Build history of the part. All positions in model axes, mm. A direction names the side the tool comes from. Give positions to 0.01 mm unless a question says otherwise; leave off trailing zeros. Loops run counter-clockwise (first coordinate to the right, second up) from the corner with the lowest first, then second, coordinate; pieces in that order, holes last. Notation, with made-up numbers: M 66,-37 L 109,-37 A14 cw 109,-23 Z; hole C 50.25,-36.75 d9. An arc over 180 degrees is marked long. Answer as a JSON object with one key per item and string values. Group by question number.
1. Slice it at B-B (x = -0.5). List the corners of the cut face in (y, z), then the cut area to 3 significant figures.
2. Slice it at C-C (y = 65). List the corners of the cut face in (x, z).
3. 3-axis set-ups, long thin cutter, end or side, ignore diameter. For faces 1 (the face through (-13, -1, 0)), 2 (the face through (86.355, 28, 36)): which of +Z, -Z, +X, -X, +Y, -Y reach the whole face in a straight line?
4. Mould opens along Y. For faces 3 (the face through (-109.645, 28, 36)), 4 (the face through (88.355, -4, 35)), 5 (the face through (-13, -102.661, 35)) say: released by +Y, released by -Y, zero draft, split by the parting line, or undercut.
5. Slice it at A-A (z = 32). List the corners of the cut face in (x, y).
6. Drill centre lines: line 1 along Y through (x, z) = (23, 8.5); line 2 along X through (y, z) = (-80, 34); line 3 along X through (y, z) = (42.5, 31). Where is each one in solid material? Low to high. Write a range as [from, to].
7. Drop a flat-ended pin along its axis: pin 1 Ø15 at (x, y) = (-8.5, 24) entering from +Z. Give the stop position or say it passes through.
from build123d import *

# Parameters (mm, degrees)
F0_W     = 200
F0_H     = 200
F1_DEPTH = 70
F2_T     = -2
F3_W     = 196
F3_H     = 2
F3_W_2   = 2
F3_H_2   = 50
F4_DEPTH = 68


with BuildPart() as f1:
    # F0 (on Top) → F1 (new body)
    with BuildSketch(Plane.XY):
        with Locations((-11.6452798247, -2.6608344432)):
            Rectangle(F0_W, F0_H)
    extrude(amount=F1_DEPTH)

    # F2
    f2_openings = [f1.faces().sort_by_distance(p)[0] for p in [
        (-11.64528, -2.660834, 70),
    ]]
    offset(amount=F2_T, openings=f2_openings)

    # F3 (on face) → F4 (join)
    with BuildSketch(Plane.XY.offset(2)):
        with Locations((-11.6452798247, 54.3391655568)):
            Rectangle(F3_W, F3_H)
        with Locations((-11.6452798247, 2.3391655568)):
            Rectangle(F3_W, F3_H)
        Polygon((86.3547201753, -48.6608344432), (-109.6452798247, -48.6608344432), (-109.6452798247, -50.6608344432), (-12.6452798247, -50.6608344432), (-10.6452798247, -50.6608344432), (86.3547201753, -50.6608344432), align=None)
        with Locations((-11.6452798247, -75.6608344432)):
            Rectangle(F3_W_2, F3_H_2)
    extrude(amount=F4_DEPTH)


solid = f1.part
Established:
{
 "1": {"outline": "M -102.66,0 L 97.34,0 L 97.34,70 L 95.34,70 L 95.34,2 L 55.34,2 L 55.34,70 L 53.34,70 L 53.34,2 L 3.34,2 L 3.34,70 L 1.34,70 L 1.34,2 L -48.66,2 L -48.66,70 L -50.66,70 L -50.66,2 L -100.66,2 L -100.66,70 L -102.66,70 Z", "area": "1,080 mm^2"},
 "2": {"outline": "M -111.65,0 L 88.35,0 L 88.35,70 L 86.35,70 L 86.35,2 L -109.65,2 L -109.65,70 L -111.65,70 Z"},
 "3": {"face 1": "-Z, +X, -X, +Y, -Y", "face 2": "+Z"},
 "4": {"face 3": "undercut", "face 4": "zero draft", "face 5": "released by -Y"},
 "5": {"outline": "M -111.65,-102.66 L 88.35,-102.66 L 88.35,97.34 L -111.65,97.34 Z; hole M -109.65,-100.66 L -12.65,-100.66 L -12.65,-50.66 L -109.65,-50.66 Z; hole M -109.65,-48.66 L 86.35,-48.66 L 86.35,1.34 L -109.65,1.34 Z; hole M -109.65,3.34 L 86.35,3.34 L 86.35,53.34 L -109.65,53.34 Z; hole M -109.65,55.34 L 86.35,55.34 L 86.35,95.34 L -109.65,95.34 Z; hole M -10.65,-100.66 L 86.35,-100.66 L 86.35,-50.66 L -10.65,-50.66 Z"},
 "6": {"line 1": "y = [-102.66, -100.66], [-50.66, -48.66], [1.34, 3.34], [53.34, 55.34], [95.34, 97.34]", "line 2": "x = [-111.65, -109.65], [-12.65, -10.65], [86.35, 88.35]", "line 3": "x = [-111.65, -109.65], [86.35, 88.35]"},
 "7": {"pin 1": "stops at z = 2"}
}
